from build123d import *

# Parameters (mm, degrees)
F1_DEPTH      = 5
F3_SIZE       = 1
F2_W          = 4.5
F2_H          = 12.5
F4_DEPTH      = 10
F5_SIZE       = 2.5
F6_R          = 1
F7_DEPTH      = 39.5010001
F8_R          = 39.5864097355
F8_R_2        = 17.5
F9_DEPTH      = 25
F10_R         = 3.4
F11_DEPTH     = 25
F13_DEPTH     = 5
F14_T4_DEPTH  = 32.2598396724
F14_S5_R      = 17.5
F14_T6_DEPTH  = 18
F14_T10_DEPTH = 32.2598396724
F14_S11_R     = 17.5
F14_T12_DEPTH = 18
F14_T16_DEPTH = 32.2598396724
F14_S17_R     = 17.5
F14_T18_DEPTH = 18
F14_T22_DEPTH = 32.2598396724
F14_S23_R     = 17.5
F14_T24_DEPTH = 18
F15_R         = 1


# Not quite as in the source:
# - a fillet or chamfer that OpenCascade refuses, or shapes differently, is made with other operations: its cross-section is extruded or revolved along the edge and cut away or added


with BuildPart() as f1:
    # F0 (on Top) → F1 (new body)
    with BuildSketch(Plane.XY):
        with BuildLine():
            ThreePointArc((19.8625961196, -15.8301909188), (23.6080012184, -12.5093598908), (25, -7.7012087429))
            Line((25, -7.7012087429), (25, 7.7012087429))
            ThreePointArc((25, 7.7012087429), (23.6080012184, 12.5093598908), (19.8625961196, 15.8301909188))
            add(Edge.make_bspline(
                [(19.8625961196, 15.8301909188), (0, 25.2681728257), (-19.8625961196, 15.8301909188)],
                knots=[0.9132750433, 0.9132750433, 0.9132750433, 2.2283176103, 2.2283176103, 2.2283176103], degree=2, weights=[1, 0.7915095459, 1]))
            ThreePointArc((-19.8625961196, 15.8301909188), (-23.6080012184, 12.5093598908), (-25, 7.7012087429))
            Line((-25, 7.7012087429), (-25, -7.7012087429))
            ThreePointArc((-25, -7.7012087429), (-23.6080012184, -12.5093598908), (-19.8625961196, -15.8301909188))
            add(Edge.make_bspline(
                [(-19.8625961196, -15.8301909188), (0, -25.2681728257), (19.8625961196, -15.8301909188)],
                knots=[4.0548676969, 4.0548676969, 4.0548676969, 5.3699102639, 5.3699102639, 5.3699102639], degree=2, weights=[1, 0.7915095459, 1]))
        make_face()
    extrude(amount=F1_DEPTH)

    # F3
    f3_edges = [f1.edges().sort_by_distance(p)[0] for p in [
        (4e-06, -20, 0),
    ]]
    chamfer(f3_edges, length=F3_SIZE)

    # F2 (on face) → F4 (join)
    with BuildSketch(Plane(origin=(0, 0, 0), x_dir=(1, 0, 0), z_dir=(0, 0, -1))):
        with Locations((12.25, 0)):
            Rectangle(F2_W, F2_H)
        with Locations((-12.25, 0)):
            Rectangle(F2_W, F2_H)
    extrude(amount=F4_DEPTH)

    # F5
    f5_edges = [f1.edges().sort_by_distance(p)[0] for p in [
        (-12.25, -6.25, -10),
        (12.25, -6.25, -10),
        (-12.25, 6.25, -10),
        (12.25, 6.25, -10),
    ]]
    chamfer(f5_edges, length=F5_SIZE)

    # F6 (on face) → F7 (cut, through all)
    with BuildSketch(Plane.YZ.offset(14.5)):
        with Locations((0, -5)):
            Circle(F6_R)
    extrude(amount=-F7_DEPTH, mode=Mode.SUBTRACT)

    # F8 (on face) → F9 (cut)
    with BuildSketch(Plane.XY.offset(5)):
        Circle(F8_R)
        with BuildLine():
            add(Edge.make_bspline(
                [(-19.8625961196, -15.8301909188), (0, -25.2681728257), (19.8625961196, -15.8301909188)],
                knots=[4.0548676969, 4.0548676969, 4.0548676969, 5.3699102639, 5.3699102639, 5.3699102639], degree=2, weights=[1, 0.7915095459, 1]))
            ThreePointArc((-19.8625961196, -15.8301909188), (-23.6080012184, -12.5093598908), (-25, -7.7012087429))
            Line((-25, -7.7012087429), (-25, 7.7012087429))
            ThreePointArc((-25, 7.7012087429), (-23.6080012184, 12.5093598908), (-19.8625961196, 15.8301909188))
            add(Edge.make_bspline(
                [(19.8625961196, 15.8301909188), (0, 25.2681728257), (-19.8625961196, 15.8301909188)],
                knots=[0.9132750433, 0.9132750433, 0.9132750433, 2.2283176103, 2.2283176103, 2.2283176103], degree=2, weights=[1, 0.7915095459, 1]))
            ThreePointArc((19.8625961196, 15.8301909188), (23.6080012184, 12.5093598908), (25, 7.7012087429))
            Line((25, 7.7012087429), (25, -7.7012087429))
            ThreePointArc((25, -7.7012087429), (23.6080012184, -12.5093598908), (19.8625961196, -15.8301909188))
        make_face(mode=Mode.SUBTRACT)
        with BuildLine():
            ThreePointArc((-25, -7.7012087429), (-23.6080012184, -12.5093598908), (-19.8625961196, -15.8301909188))
            add(Edge.make_bspline(
                [(-19.8625961196, -15.8301909188), (0, -25.2681728257), (19.8625961196, -15.8301909188)],
                knots=[4.0548676969, 4.0548676969, 4.0548676969, 5.3699102639, 5.3699102639, 5.3699102639], degree=2, weights=[1, 0.7915095459, 1]))
            ThreePointArc((19.8625961196, -15.8301909188), (23.6080012184, -12.5093598908), (25, -7.7012087429))
            Line((25, -7.7012087429), (25, 7.7012087429))
            ThreePointArc((25, 7.7012087429), (23.6080012184, 12.5093598908), (19.8625961196, 15.8301909188))
            add(Edge.make_bspline(
                [(19.8625961196, 15.8301909188), (0, 25.2681728257), (-19.8625961196, 15.8301909188)],
                knots=[0.9132750433, 0.9132750433, 0.9132750433, 2.2283176103, 2.2283176103, 2.2283176103], degree=2, weights=[1, 0.7915095459, 1]))
            ThreePointArc((-19.8625961196, 15.8301909188), (-23.6080012184, 12.5093598908), (-25, 7.7012087429))
            Line((-25, 7.7012087429), (-25, -7.7012087429))
        make_face()
        Circle(F8_R_2, mode=Mode.SUBTRACT)
    extrude(amount=-F9_DEPTH, mode=Mode.SUBTRACT)

    # F10 (on face) → F11 (cut)
    with BuildSketch(Plane.XY.offset(5)):
        Circle(F10_R)
    extrude(amount=-F11_DEPTH, mode=Mode.SUBTRACT)

    # F12 (on face) → F13 (join)
    with BuildSketch(Plane(origin=(0, 0, 0), x_dir=(1, 0, 0), z_dir=(0, 0, -1))):
        with BuildLine():
            Line((-17.5, 12), (-17.5, -1.86e-08))
            ThreePointArc((-17.5, -1.86e-08), (-16.2659219885, 6.4552135413), (-12.7377392029, 12))
            Line((-12.7377392029, 12), (-17.5, 12))
        make_face()
        with BuildLine():
            ThreePointArc((12.7377392029, 12), (16.2659219851, 6.4552135499), (17.5, 0))
            Line((17.5, 0), (17.5, 12))
            Line((17.5, 12), (12.7377392029, 12))
        make_face()
        with BuildLine():
            Line((12.7377392029, -12), (17.5, -12))
            Line((17.5, -12), (17.5, 0))
            ThreePointArc((17.5, 0), (16.2659219851, -6.4552135499), (12.7377392029, -12))
        make_face()
        with BuildLine():
            Line((-17.5, -12), (-12.7377392029, -12))
            ThreePointArc((-12.7377392029, -12), (-16.2659219817, -6.4552135586), (-17.5, -1.86e-08))
            Line((-17.5, -1.86e-08), (-17.5, -12))
        make_face()
    extrude(amount=-F13_DEPTH)

    # F14: chamfer of 5.3 on 4 edges, made by hand


with BuildPart() as f14_tool2:
    # F14_s3 → F14_t4 (new body)
    with BuildSketch(Plane.XY.offset(-13.6299198362)):
        Polygon((17.5, -6.7), (12.2, -12), (17.5, -12), align=None)
    extrude(amount=F14_T4_DEPTH)

    # F14_s5 → F14_t6 (cut, symmetric)
    with BuildSketch(Plane.XY.offset(2.5)):
        Circle(F14_S5_R)
    extrude(amount=F14_T6_DEPTH, both=True, mode=Mode.SUBTRACT)


with BuildPart() as f1_1:
    add(f1.part)

    # F14_t1: cut F14_tool2
    add(f14_tool2.part, mode=Mode.SUBTRACT)


with BuildPart() as f14_tool8:
    # F14_s9 → F14_t10 (new body)
    with BuildSketch(Plane.XY.offset(-13.6299198362)):
        Polygon((12.2, 12), (17.5, 6.7), (17.5, 12), align=None)
    extrude(amount=F14_T10_DEPTH)

    # F14_s11 → F14_t12 (cut, symmetric)
    with BuildSketch(Plane.XY.offset(2.5)):
        Circle(F14_S11_R)
    extrude(amount=F14_T12_DEPTH, both=True, mode=Mode.SUBTRACT)


with BuildPart() as f1_2:
    add(f1_1.part)

    # F14_t7: cut F14_tool8
    add(f14_tool8.part, mode=Mode.SUBTRACT)


with BuildPart() as f14_tool14:
    # F14_s15 → F14_t16 (new body)
    with BuildSketch(Plane.XY.offset(-13.6299198362)):
        Polygon((-12.2, -12), (-17.5, -6.7), (-17.5, -12), align=None)
    extrude(amount=F14_T16_DEPTH)

    # F14_s17 → F14_t18 (cut, symmetric)
    with BuildSketch(Plane.XY.offset(2.5)):
        Circle(F14_S17_R)
    extrude(amount=F14_T18_DEPTH, both=True, mode=Mode.SUBTRACT)


with BuildPart() as f1_3:
    add(f1_2.part)

    # F14_t13: cut F14_tool14
    add(f14_tool14.part, mode=Mode.SUBTRACT)


with BuildPart() as f14_tool20:
    # F14_s21 → F14_t22 (new body)
    with BuildSketch(Plane.XY.offset(-13.6299198362)):
        Polygon((-17.5, 6.7), (-12.2, 12), (-17.5, 12), align=None)
    extrude(amount=F14_T22_DEPTH)

    # F14_s23 → F14_t24 (cut, symmetric)
    with BuildSketch(Plane.XY.offset(2.5)):
        Circle(F14_S23_R)
    extrude(amount=F14_T24_DEPTH, both=True, mode=Mode.SUBTRACT)


with BuildPart() as f1_4:
    add(f1_3.part)

    # F14_t19: cut F14_tool20
    add(f14_tool20.part, mode=Mode.SUBTRACT)

    # F15
    f15_edges = [f1_4.edges().sort_by_distance(p)[0] for p in [
        (-17.5, -6.7, 2.5),
        (-17.5, 6.7, 2.5),
        (17.5, 6.7, 2.5),
        (17.5, -6.7, 2.5),
    ]]
    fillet(f15_edges, radius=F15_R)


solid = f1_4.part
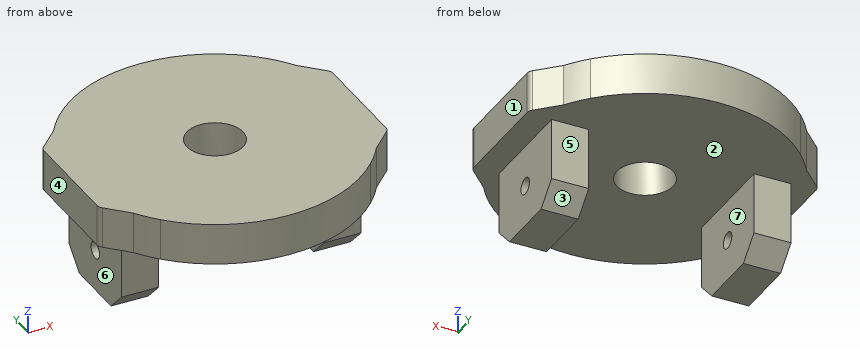
Here's how the part is built. I have some questions about the finished solid (model axes, mm). Face numbers are marked on the shaded views. A direction names the side the tool comes from. Coordinates: 2 decimals unless noted, no trailing zeros. Order: outer loops, then holes, each group sorted by start corner. A loop starts at its lowest first (then second) coordinate and runs counter-clockwise, first axis right, second up. Notation, with made-up numbers: M -10,-13 L -5,-13 A32 cw -5,24 Z; hole C 64.25,9.5 d1. An arc over 180 degrees is marked long. Answer as CSV lines item,"result".
Item 1: Imagine slicing it at C-C on y = 0. Write out the boundary of the cut face in (x, z), plus the area to 3 significant figures.
Results found:
outline,"M -17.5,0 L -14.5,0 L -14.5,-4 L -10,-4 L -10,0 L -3.4,0 L -3.4,5 L -17.5,5 Z; M -14.5,-10 L -10,-10 L -10,-6 L -14.5,-6 Z; M 3.4,0 L 10,0 L 10,-4 L 14.5,-4 L 14.5,0 L 17.5,0 L 17.5,5 L 3.4,5 Z; M 10,-10 L 14.5,-10 L 14.5,-6 L 10,-6 Z"
area,"213 mm2"
Item 2: For pin 1 (5 mm diameter, centred on y = -1.5, z = -7, fed in from -X); pin 2 (4 mm diameter, centred on x = -3, y = -7.5, fed in from -Z); pin 3 (2 mm diameter, centred on x = 12.5, z = -4, fed in from -Y); pin 4 (1.2 mm diameter, centred on y = 0, z = -5, fed in from -X), each with a flat end and sliding along its axis, tell me the tip position at first contact or that it passes through.
Results found:
pin 1,"x = -14.5"
pin 2,"z = 0"
pin 3,"y = -6.25"
pin 4,"through"
Item 3: Imagine slicing it at A-A on z = -5. Write out the boundary of the cut face in (x, y), plus the area to 3 significant figures.
Results found:
outline,"M -14.5,-6.25 L -10,-6.25 L -10,-1 L -14.5,-1 Z; M -14.5,1 L -10,1 L -10,6.25 L -14.5,6.25 Z; M 10,-6.25 L 14.5,-6.25 L 14.5,-1 L 10,-1 Z; M 10,1 L 14.5,1 L 14.5,6.25 L 10,6.25 Z"
area,"94.5 mm2"
Item 4: Imagine slicing it at B-B on x = 0. Write out the boundary of the cut face in (y, z), plus the area to 3 significant figures.
Results found:
outline,"M -17.5,0 L -3.4,0 L -3.4,5 L -17.5,5 Z; M 3.4,0 L 17.5,0 L 17.5,5 L 3.4,5 Z"
area,"141 mm2"
Item 5: Imagine slicing it at D-D on x = -14. Write out the boundary of the cut face in (y, z).
Results found:
outline,"M -10.5,0 L -6.25,0 L -6.25,-7.5 L -3.75,-10 L 3.75,-10 L 6.25,-7.5 L 6.25,0 L 10.5,0 L 10.5,5 L -10.5,5 Z; hole C 0,-5 d2"
Item 6: If I drill on line 1 (Z direction, x = -12.8, y = 0); line 2 (Y direction, x = 0, z = 2.05); line 3 (Z direction, x = 4, y = -16), over which ranges is the centre line in solid material (lowest first)?
Results found:
line 1,"-10 to -6, -4 to 5"
line 2,"-17.5 to -3.4, 3.4 to 17.5"
line 3,"0 to 5"
Item 7: We'd pull the mould along X, two halves only. Please class the marked faces 1, 2, 3 and 4: +X half, -X half, draft (parallel to the pull), parting line (faces both ways), or undercut.
Results found:
face 1,"+X half"
face 2,"undercut"
face 3,"draft"
face 4,"-X half"
Item 8: On a 3-axis mill with a long thin cutter (end or side, diameter ignored), from which of +Z, -Z, +X, -X, +Y, -Y can I reach the whole of each face in a straight line? I mean the marked faces 5, 6 and 7. Say none if no direction works.
Results found:
face 5,"-Z, +X, -X, +Y"
face 6,"-Z, -X, +Y, -Y"
face 7,"-Z, +Y, -Y"
